Can you work these out from the model? Positions are in its coordinate system, mm. Face numbers are marked on the shaded views. A direction names the side the tool comes from. Give positions to 0.01 mm unless a question says otherwise; leave off trailing zeros. Order: outer loops, then holes, each group sorted by start corner. A loop starts at its lowest first (then second) coordinate and runs counter-clockwise, first axis right, second up. Notation, with made-up numbers: (-1, 74) -> (53, 74) arc R21 ccw to (53, 107) -> close; hole circle Ø3 at (32, 86.5). An arc over 180 degrees is marked (long way). Answer as CSV lines item,"result".
```python
from build123d import *

# Parameters (mm, degrees)
F0_R      = 16.51
F0_R_2    = 12.7
F1_DEPTH  = 76.2
F1_FACE_R = 16.51
F2_DEPTH  = 25.4
F2_TAPER  = 35
F4_DEPTH  = 2.54
F5_COUNT  = 4
F6_R      = 11.43
F7_DEPTH  = 73.914


with BuildPart() as f1:
    # F0 (on Top) → F1 (new body)
    with BuildSketch(Plane.XY):
        Circle(F0_R)
        Circle(F0_R_2, mode=Mode.SUBTRACT)
        Circle(F0_R_2)
    extrude(amount=F1_DEPTH)

    # F1_face (on face) → F2 (join)
    with BuildSketch(Plane.XY.offset(76.2)):
        Circle(F1_FACE_R)
    extrude(amount=F2_DEPTH, taper=F2_TAPER)

    # F3 (on Right) → F4 (join, symmetric)
    with BuildSketch(Plane.YZ):
        Polygon((-40.5384004116, 0), (-15.8495996147, 0), (-15.8495996147, 18.7452007085), align=None)
    extrude(amount=F4_DEPTH, both=True)

    # F5: F1 ×4 about axis
    f5_axis = Axis((0, 0, 76.2), (0, 0, 1))


with BuildPart() as f1_1:
    add(f1.part)
    for i in range(1, F5_COUNT):
        add(f1.part.rotate(f5_axis, i * 360 / F5_COUNT))

    # F6 (on face) → F7 (cut)
    with BuildSketch(Plane(origin=(0, 0, 0), x_dir=(1, 0, 0), z_dir=(0, 0, -1))):
        Circle(F6_R)
    extrude(amount=-F7_DEPTH, mode=Mode.SUBTRACT)


solid = f1_1.part
```
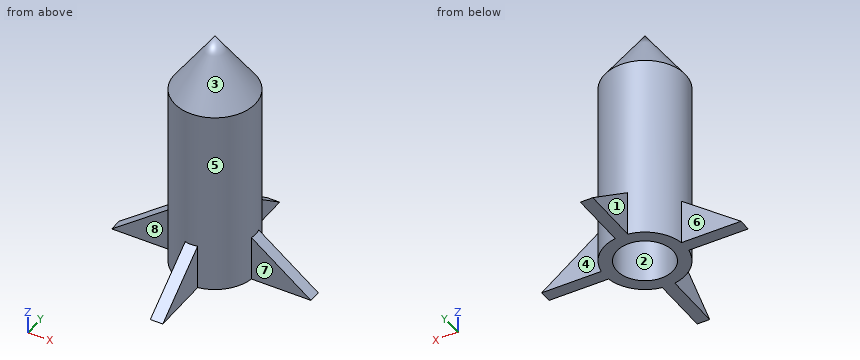
Item 1: Imagine slicing it at C-C, the plane z = 11. Please give me the cut outline in (x, y).
Numbers:
outline,"(-26.05, -2.54) -> (-16.31, -2.54) arc R16.51 ccw to (-2.54, -16.31) -> (-2.54, -26.05) -> (2.54, -26.05) -> (2.54, -16.31) arc R16.51 ccw to (16.31, -2.54) -> (26.05, -2.54) -> (26.05, 2.54) -> (16.31, 2.54) arc R16.51 ccw to (2.54, 16.31) -> (2.54, 26.05) -> (-2.54, 26.05) -> (-2.54, 16.31) arc R16.51 ccw to (-16.31, 2.54) -> (-26.05, 2.54) -> close; hole circle Ø22.86 at (0, 0)"
Item 2: Imagine slicing it at B-B, the plane x = 19.5. Please give me the cut outline in (y, z).
Numbers:
outline,"(-2.54, 0) -> (2.54, 0) -> (2.54, 15.97) -> (-2.54, 15.97) -> close"
Item 3: Imagine slicing it at D-D, the plane z = 81.5. Please give me the cut outline in (x, y), then the cut area to 3 significant figures.
Numbers:
outline,"circle Ø25.6 at (0, 0)"
area,"515 mm²"
Item 4: We'd pull the mould along X, two halves only. Please class the marked faces 1, 2, 3 and 4: released by +X, released by -X, zero draft, split by the parting line, or undercut.
Numbers:
face 1,"released by -X"
face 2,"undercut"
face 3,"split by the parting line"
face 4,"zero draft"
Item 5: Please list where these lines run through material, in increasing order: line 1 along Y through (x, z) = (0, 30); line 2 along Y through (x, z) = (30.5, 6).
Numbers:
line 1,"y = -16.51 to -11.43, 11.43 to 16.51"
line 2,"y = -2.54 to 2.54"
Item 6: For pin 1 (20 mm diameter, centred on x = -26.5, z = 9, fed in from +Y); pin 2 (5 mm diameter, centred on x = -5, y = -26.5, fed in from -Z); pin 3 (20 mm diameter, centred on y = 32, z = 11.5, fed in from +X); pin 4 (12 mm diameter, centred on x = 1, y = 23, fed in from +Z), each with a flat end and sliding along its axis, tell me the tip position at first contact or that it passes through.
Numbers:
pin 1,"stops at y = 2.54"
pin 2,"stops at z = 0"
pin 3,"stops at x = 2.54"
pin 4,"stops at z = 17.87"
Item 7: For the marked faces 5, 6, 7 and 8, which set-ups out of +Z, -Z, +X, -X, +Y, -Y let a thin tool reach every point of the face, with its end or its side?
Numbers:
face 5,"+Z"
face 6,"+Z, -Z, -X, +Y"
face 7,"+Z, -Z, +X, -Y"
face 8,"+Z, -Z, -X, -Y"
Item 8: Imagine slicing it at A-A, the plane z = 22.5. Please give me the cut outline in (x, y), then the cut area to 3 significant figures.
Numbers:
outline,"circle Ø33.02 at (0, 0); hole circle Ø22.86 at (0, 0)"
area,"446 mm²"
